Read the model definition and answer for the solid it produces. Units are mm, in the model's axes. Face numbers are marked on the shaded views. A direction names the side the tool comes from. Give positions to 0.01 mm unless a question says otherwise; leave off trailing zeros. Loops run counter-clockwise (first coordinate to the right, second up) from the corner with the lowest first, then second, coordinate; pieces in that order, holes last. Notation, with made-up numbers: (-4, -25) -> (55, -25) arc R18 ccw to (55, -15) -> close; hole circle Ø4 at (-29.75, -4.75). An arc over 180 degrees is marked (long way). One line per item, written item: value. Start each with the question number.
from build123d import *

# Parameters (mm, degrees)
BODY_DEPTH     = 60
SK_FINGER_A_W  = 20
SK_FINGER_A_H  = 10
FINGER_A_DEPTH = 54
SK_FINGER_B_W  = 20
SK_FINGER_B_H  = 10
FINGER_B_DEPTH = 54


with BuildPart() as part:
    # SK_Body → Body (new body)
    with BuildSketch(Plane.XY.offset(-66)):
        Polygon((-24, -22), (24, -22), (30, -16), (30, 16), (24, 22), (-24, 22), (-30, 16), (-30, -16), align=None)
    extrude(amount=BODY_DEPTH)

    # SK_Finger_A → Finger_A (add)
    with BuildSketch(Plane.XY.offset(-120)):
        with Locations((0, 11)):
            Rectangle(SK_FINGER_A_W, SK_FINGER_A_H)
    extrude(amount=FINGER_A_DEPTH)

    # SK_Finger_B → Finger_B (add)
    with BuildSketch(Plane.XY.offset(-120)):
        with Locations((0, -11)):
            Rectangle(SK_FINGER_B_W, SK_FINGER_B_H)
    extrude(amount=FINGER_B_DEPTH)


solid = part.part
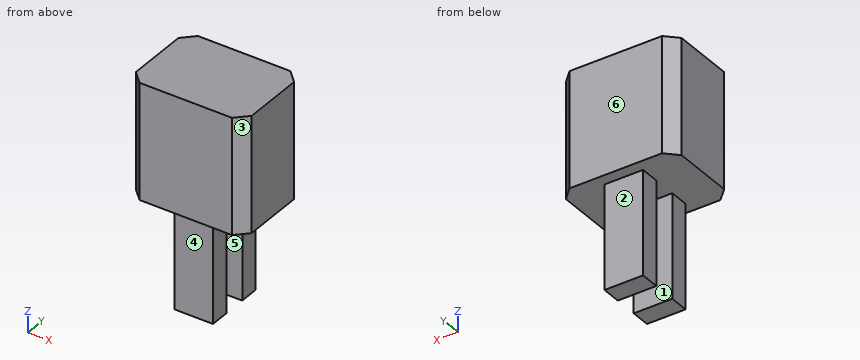
Item 1: Section B-B, the plane x = -5 is taken. Determine the outline of the cut face in (y, z).
Item 2: For the marked faces 1, 2 and 3, determine the directions among +Z, -Z, +X, -X, +Y, -Y from which every point of the face is accessible in a straight line to the end or side of a thin tool.
Item 3: Section C-C, the plane y = -9.5 is taken. Determine the outline of the cut face in (x, z).
Item 4: Flat-ended cylindrical pins translate along their axes: pin 1 (6 mm diameter, centred on x = -4.5, z = -98, fed in from +Y); pin 2 (11 mm diameter, centred on y = 9, z = -96.5, fed in from -X); pin 3 (3 mm diameter, centred on y = -12.5, z = -90.5, fed in from +X). Find the tip coordinate at first contact, or state that the pin passes through.
Item 5: Determine the mould class of the marked faces 4, 5 and 6 for opening direction Y: pulls with the +Y half, pulls with the -Y half, needs draft (parallel to the pull), parting line crosses it, or undercut.
Item 6: Section D-D, the plane z = -16 is taken. Determine the outline of the cut face in (x, y), plus the area to 3 significant figures.
Item 7: Consider L1, parallel to Y at x = -8.5, z = -115; L2, parallel to X at y = -9, z = -108; L3, parallel to Z at x = -1, y = 4.5. Determine where each line is inside the solid, lowest interval first. Write a range as [from, to].
Item 8: Section A-A, the plane z = -100.5 is taken. Determine the outline of the cut face in (x, y).
Computed values:
1. outline: (-22, -66) -> (-16, -66) -> (-16, -120) -> (-6, -120) -> (-6, -66) -> (6, -66) -> (6, -120) -> (16, -120) -> (16, -66) -> (22, -66) -> (22, -6) -> (-22, -6) -> close
2. face 1: -Z, +X, -X
2. face 2: -Z, +X, -X, +Y
2. face 3: +Z, -Z, +X, -Y
3. outline: (-30, -66) -> (-10, -66) -> (-10, -120) -> (10, -120) -> (10, -66) -> (30, -66) -> (30, -6) -> (-30, -6) -> close
4. pin 1: y = 16
4. pin 2: x = -10
4. pin 3: x = 10
5. face 4: pulls with the -Y half
5. face 5: undercut
5. face 6: pulls with the +Y half
6. outline: (-30, -16) -> (-24, -22) -> (24, -22) -> (30, -16) -> (30, 16) -> (24, 22) -> (-24, 22) -> (-30, 16) -> close
6. area: 2,570 mm²
7. L1: [-16, -6], [6, 16]
7. L2: [-10, 10]
7. L3: [-66, -6]
8. outline: (-10, -16) -> (10, -16) -> (10, -6) -> (-10, -6) -> close; (-10, 6) -> (10, 6) -> (10, 16) -> (-10, 16) -> close
